```python
from build123d import *

# Parameters (mm, degrees)
CYLINDER003_R     = 1.4
CYLINDER003_DEPTH = 2
CYLINDER001_R     = 1.4
CYLINDER001_DEPTH = 2
CYLINDER002_R     = 1.4
CYLINDER002_DEPTH = 2
CYLINDER_R        = 1.4
CYLINDER_DEPTH    = 2
BOX_W             = 134
BOX_H             = 53
BOX_DEPTH         = 2
FILLET_R          = 2


with BuildPart() as cylinder003:
    # Cylinder003 → Cylinder003 (new body)
    with BuildSketch(Plane(origin=(130.4, 48, 0), x_dir=(1, 0, 0), z_dir=(0, 0, 1))):
        Circle(CYLINDER003_R)
    extrude(amount=CYLINDER003_DEPTH)


with BuildPart() as cylinder001:
    # Cylinder001 → Cylinder001 (new body)
    with BuildSketch(Plane(origin=(3.8, 48, 0), x_dir=(1, 0, 0), z_dir=(0, 0, 1))):
        Circle(CYLINDER001_R)
    extrude(amount=CYLINDER001_DEPTH)


with BuildPart() as cylinder002:
    # Cylinder002 → Cylinder002 (new body)
    with BuildSketch(Plane(origin=(130.4, 2.97, 0), x_dir=(1, 0, 0), z_dir=(0, 0, 1))):
        Circle(CYLINDER002_R)
    extrude(amount=CYLINDER002_DEPTH)


with BuildPart() as fusion:
    # Cylinder → Cylinder (new body)
    with BuildSketch(Plane(origin=(3.8, 2.97, 0), x_dir=(1, 0, 0), z_dir=(0, 0, 1))):
        Circle(CYLINDER_R)
    extrude(amount=CYLINDER_DEPTH)

    # Fusion: union Cylinder003, Cylinder001, Cylinder002
    add(cylinder003.part)
    add(cylinder001.part)
    add(cylinder002.part)


with BuildPart() as cut:
    # Box → Box (new body)
    with BuildSketch(Plane.XY):
        with Locations((67, 26.5)):
            Rectangle(BOX_W, BOX_H)
    extrude(amount=BOX_DEPTH)

    # Fillet
    fillet_edges = [cut.edges().sort_by_distance(p)[0] for p in [
        (0, 53, 1),
        (134, 53, 1),
    ]]
    fillet(fillet_edges, radius=FILLET_R)

    # Cut: cut Fusion
    add(fusion.part, mode=Mode.SUBTRACT)


solid = cut.part
```
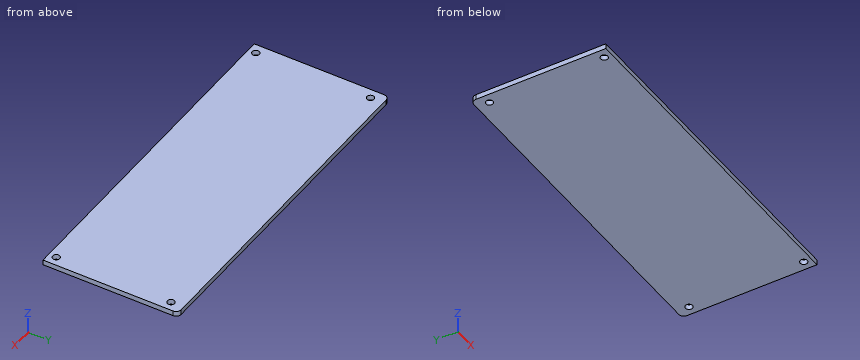
Part model, mm, in its own coordinate system. Round coordinates to 2 decimals unless told otherwise and drop trailing zeros. Write each loop counter-clockwise with the first axis right and the second up, starting at its lowest first coordinate (ties: lowest second). Pieces come first, ordered by that corner, then holes. Notation, with made-up numbers: (89.25, 17) -> (140.25, 17) arc R10 cw to (140.25, 35) -> close; hole circle Ø7 at (82, 76). An arc over 180 degrees is marked (long way). Return JSON: item names as keys, results as strings. Group by question number.
Q1. Saw through at B-B on x = 130.4. Write the cut outline in (y, z), plus the area to 3 significant figures.
Q2. Saw through at A-A on y = 48. Write the cut outline in (x, z), plus the area to 3 significant figures.
Q3. Pin check, flat tips, straight feed: pin 1 (3.5 mm diameter, centred on x = 130.4, y = 2.97, fed in from -Z); pin 2 (2 mm diameter, centred on x = 130.4, y = 48, fed in from +Z). Stop position of each tip, or through.
Q4. Probe L1, parallel to Y at x = 130.4, z = 1.25; L2, parallel to X at y = 47.5, z = 0.65. List the from-to ranges inside material, lowest first. Write a range as [from, to].
Answer:
{
 "1": {"outline": "(0, 0) -> (1.57, 0) -> (1.57, 2) -> (0, 2) -> close; (4.37, 0) -> (46.6, 0) -> (46.6, 2) -> (4.37, 2) -> close; (49.4, 0) -> (53, 0) -> (53, 2) -> (49.4, 2) -> close", "area": "94.8 mm2"},
 "2": {"outline": "(0, 0) -> (2.4, 0) -> (2.4, 2) -> (0, 2) -> close; (5.2, 0) -> (129, 0) -> (129, 2) -> (5.2, 2) -> close; (131.8, 0) -> (134, 0) -> (134, 2) -> (131.8, 2) -> close", "area": "257 mm2"},
 "3": {"pin 1": "z = 0", "pin 2": "through"},
 "4": {"L1": "[0, 1.57], [4.37, 46.6], [49.4, 53]", "L2": "[0, 2.49], [5.11, 129.09], [131.71, 134]"}
}
